Design review of the part built by this model. Coordinates are the model's own, in mm. Face numbers are marked on the shaded views. Coordinates: 2 decimals unless noted, no trailing zeros. Write each loop counter-clockwise with the first axis right and the second up, starting at its lowest first coordinate (ties: lowest second). Pieces come first, ordered by that corner, then holes.
Q1. Take a section at A-A, the plane z = 17.25. Write out the cut boundary in (x, y).
Q2. The part is to be moulded in two halves that separate along Z. For the marked faces 1, 2 and 3, say which applies: released by +Z, released by -Z, zero draft, split by the parting line, or undercut.
Q3. For L1, parallel to X at y = 3.45, z = 12.7; L2, parallel to X at y = -2.5, z = 12.7; L3, parallel to Z at x = -15.5, y = -7.5, list the stretches that pass through material, from the lowest coordinate up.
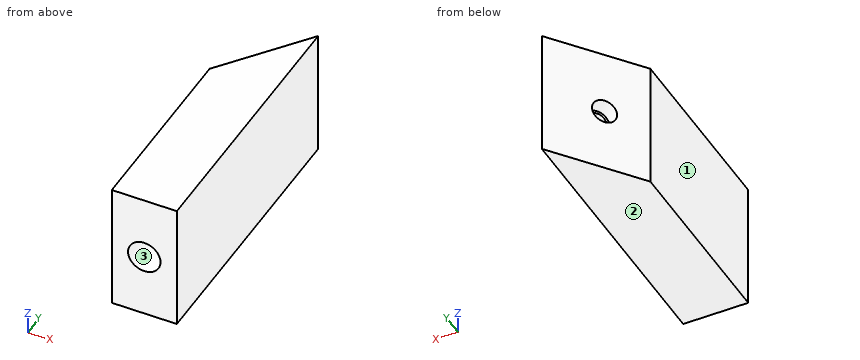
from build123d import *

# Parameters (mm, degrees)
EXTRUDE1_DEPTH                    = 25.4
F_1_4_20_TAPPED_HOLE3_D           = 5.1054
F_1_4_20_TAPPED_HOLE3_DEPTH       = 16.51
F_1_4_20_TAPPED_HOLE3_CBORE_D     = 6.35
F_1_4_20_TAPPED_HOLE3_CBORE_DEPTH = 12.7
F_1_4_20_TAPPED_HOLE3_TIP         = 1.533816902
F_10_24_TAPPED_HOLE1_D            = 3.7973
F_10_24_TAPPED_HOLE1_DEPTH        = 6.35
F_10_24_TAPPED_HOLE1_CBORE_D      = 4.826
F_10_24_TAPPED_HOLE1_CBORE_DEPTH  = 3.175
F_10_24_TAPPED_HOLE1_TIP          = 1.140824014


with BuildPart() as part:
    # Sketch1 → Extrude1 (new body)
    with BuildSketch(Plane.XY):
        Polygon((-8.815807595, 41.879239751), (-21.52120708, 25.279287896), (-21.52120708, -11.990787033), (-8.815807595, -11.990787033), align=None)
    extrude(amount=EXTRUDE1_DEPTH)

    # 1/4-20 Tapped Hole3
    with Locations(Plane(origin=(6.946606398, -11.990787033, 18.061260674), x_dir=(-1, 0, 0), z_dir=(0, -1, 0))):
        with Locations((22.117813477, 5.361260674)):
            CounterBoreHole(F_1_4_20_TAPPED_HOLE3_D / 2, F_1_4_20_TAPPED_HOLE3_CBORE_D / 2, F_1_4_20_TAPPED_HOLE3_CBORE_DEPTH, depth=F_1_4_20_TAPPED_HOLE3_DEPTH)
            with Locations((0, 0, -(F_1_4_20_TAPPED_HOLE3_DEPTH + F_1_4_20_TAPPED_HOLE3_TIP / 2))):  # 118° drill point
                Cone(0, F_1_4_20_TAPPED_HOLE3_D / 2, F_1_4_20_TAPPED_HOLE3_TIP, mode=Mode.SUBTRACT)

    # #10-24 Tapped Hole1
    with Locations(Plane(origin=(13.322416251, 70.803434574, 18.061260674), x_dir=(0.6077917109686657, 0.794096490407672, 0), z_dir=(-0.794096490407672, 0.6077917109686657, 0))):
        with Locations((-48.503844205, 5.361260674)):
            CounterBoreHole(F_10_24_TAPPED_HOLE1_D / 2, F_10_24_TAPPED_HOLE1_CBORE_D / 2, F_10_24_TAPPED_HOLE1_CBORE_DEPTH, depth=F_10_24_TAPPED_HOLE1_DEPTH)
            with Locations((0, 0, -(F_10_24_TAPPED_HOLE1_DEPTH + F_10_24_TAPPED_HOLE1_TIP / 2))):  # 118° drill point
                Cone(0, F_10_24_TAPPED_HOLE1_D / 2, F_10_24_TAPPED_HOLE1_TIP, mode=Mode.SUBTRACT)


solid = part.part
Responses:
1. outline: (-21.52, -11.99) - (-8.82, -11.99) - (-8.82, 41.88) - (-21.52, 25.28) - close
2. face 1: zero draft
2. face 2: released by -Z
2. face 3: undercut
3. L1: x = -21.52 to -17.72, -12.62 to -8.82
3. L2: x = -21.52 to -18.35, -12 to -8.82
3. L3: z = 0 to 9.54, 15.86 to 25.4
